from build123d import *

# Parameters (mm, degrees)
BOSS_EXTRUDE1_DEPTH = 12.7


with BuildPart() as part:
    # Sketch1 → Boss-Extrude1 (new body)
    with BuildSketch(Plane(origin=(0, 0, 0), x_dir=(0, 0, -1), z_dir=(1, 0, 0))):
        with BuildLine():
            Line((1.4125, 63.5), (15.875, 63.5))
            Line((15.875, 63.5), (15.875, 61.9125))
            Line((15.875, 61.9125), (3, 61.9125))
            ThreePointArc((3, 61.9125), (0.878679656, 61.033820344), (0, 58.9125))
            Line((0, 58.9125), (0, 3))
            ThreePointArc((0, 3), (-0.878679656, 0.878679656), (-3, 0))
            Line((-3, 0), (-17.4625, 0))
            Line((-17.4625, 0), (-17.4625, 1.5875))
            Line((-17.4625, 1.5875), (-4.5875, 1.5875))
            ThreePointArc((-4.5875, 1.5875), (-2.466179656, 2.466179656), (-1.5875, 4.5875))
            Line((-1.5875, 4.5875), (-1.5875, 60.5))
            ThreePointArc((-1.5875, 60.5), (-0.708820344, 62.621320344), (1.4125, 63.5))
        make_face()
    extrude(amount=BOSS_EXTRUDE1_DEPTH)


solid = part.part
The listing builds one solid part. Answer for the finished solid, in the listing's coordinates (mm). A direction names the side the tool comes from. Give positions to 0.01 mm unless a question says otherwise; leave off trailing zeros. Order: outer loops, then holes, each group sorted by start corner. A loop starts at its lowest first (then second) coordinate and runs counter-clockwise, first axis right, second up. Notation, with made-up numbers: (-29.5, 54.25) - (24.5, 54.25) arc R25 ccw to (24.5, 70.25) - close; hole circle Ø9 at (44.25, 10). An arc over 180 degrees is marked (long way). One line per item, written item: value. Start each with the question number.
1) Given pin 1 Ø6.5 at (x, z) = (4.5, 13.5) entering from +Y; pin 2 Ø3 at (x, y) = (1.5, 40.5) entering from +Z; pin 3 Ø4 at (x, y) = (9, 17.5) entering from -Z, each flat-ended and moving along its own axis, determine where each tip first touches the part or whether it passes through.
2) Find the intervals of material crossed by L1, parallel to Z at x = 10.75, y = 28; L2, parallel to Y at x = 4.5, z = -3, in increasing order.
3) A tool of negligible diameter and unlimited length cuts with its end or side. For faces 1 (the face through (6, 32, 1.588)), 2 (the face through (6, 61.912, -10)), 3 (the face through (6, 63, -15.875)), from which of +Z, -Z, +X, -X, +Y, -Y can it reach the whole face along a straight path? Write none if from no direction.
4) A cutting plane is placed at A-A on x = 10.5. Give the vertices of the cut face in (y, z) (1 decimal), then the cut area to 3 significant figures.
5) A cutting plane is placed at B-B on z = 8. Give the vertices of the cut face in (x, y).
Answer sheet:
1. pin 1: stops at y = 1.59
1. pin 2: stops at z = 1.59
1. pin 3: stops at z = 0
2. L1: z = 0 to 1.59
2. L2: y = 61.91 to 63.5
3. face 1: +Z, +X, -X, +Y
3. face 2: -Z, +X, -X, -Y
3. face 3: -Z, +X, -X, +Y, -Y
4. outline: (0, 3) arc R3 ccw to (3, 0) - (58.9, 0) arc R3 cw to (61.9, -3) - (61.9, -15.9) - (63.5, -15.9) - (63.5, -1.4) arc R3 ccw to (60.5, 1.6) - (4.6, 1.6) arc R3 cw to (1.6, 4.6) - (1.6, 17.5) - (0, 17.5) - close
4. area: 151 mm2
5. outline: (0, 0) - (12.7, 0) - (12.7, 1.59) - (0, 1.59) - close
